Print and shaded views of the part. All mm, measured from the part's lowest x, y and z. Round coordinates to 2 decimals unless told otherwise and drop trailing zeros. Loops run counter-clockwise (first coordinate to the right, second up) from the corner with the lowest first, then second, coordinate; pieces in that order, holes last. Notation, with made-up numbers: (41, 38.25) -> (74, 38.25) arc R28 ccw to (74, 66.25) -> close; hole circle Ø7 at (60, -25.5). An arc over 180 degrees is marked (long way). Answer as CSV lines item,"result".
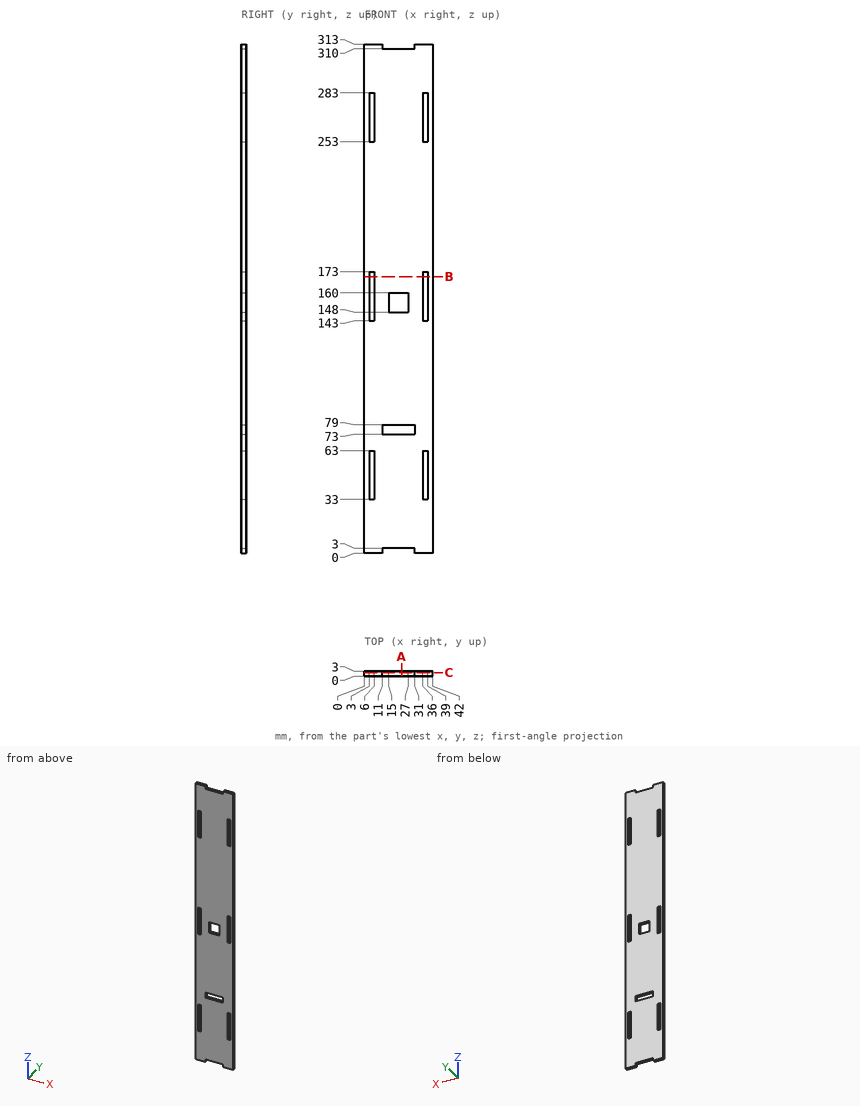
Q1. Probe L1, parallel to Z at x = 5, y = 2.4; L2, parallel to Z at x = 25, y = 0.7; L3, parallel to X at y = 1.65, z = 44. List the from-to ranges inside material, lowest first. Write a range as [from, to].
Results:
L1,"[0, 33], [63, 143], [173, 253], [283, 313]"
L2,"[3, 73], [79, 148], [160, 310]"
L3,"[0, 3], [6, 36], [39, 42]"
Q2. Slice it at A-A, the plane x = 23. Give the cut face in (y, z), and give its area (3 significant figures).
Results:
outline,"(0, 3) -> (3, 3) -> (3, 73) -> (0, 73) -> close; (0, 79) -> (3, 79) -> (3, 148) -> (0, 148) -> close; (0, 160) -> (3, 160) -> (3, 310) -> (0, 310) -> close"
area,"867 mm2"
Q3. Slice it at B-B, the plane z = 170. Give the cut face in (x, y).
Results:
outline,"(0, 0) -> (3, 0) -> (3, 3) -> (0, 3) -> close; (6, 0) -> (36, 0) -> (36, 3) -> (6, 3) -> close; (39, 0) -> (42, 0) -> (42, 3) -> (39, 3) -> close"
Q4. Slice it at C-C, the plane y = 2. Count the separate pieces of the cut face and the enclosed holes in it, and give its area (3 significant figures).
Results:
separate pieces,"1"
enclosed holes,"8"
area,"12,200 mm2"
Q5. Drop flat-ended pins along their axis: pin 1 Ø0.9 at (x, y) = (20.5, 2) entering from +Z; pin 2 Ø1 at (x, y) = (21.5, 2) entering from -Z. Give the stop position or say it passes through.
Results:
pin 1,"z = 310"
pin 2,"z = 3"
